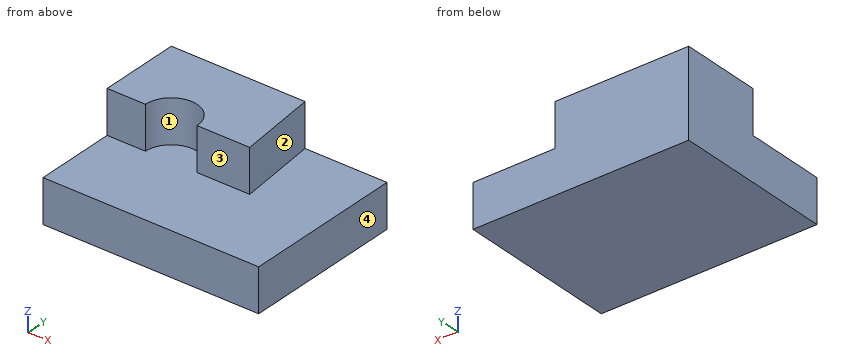
from build123d import *

# Parameters (mm, degrees)
F0_W     = 127
F0_H     = 95.25
F1_DEPTH = 25.4
F2_W     = 127
F2_H     = 47.6253371388
F3_DEPTH = 25.4
F5_DEPTH = 25.4


with BuildPart() as f1:
    # F0 (on Top) → F1 (new body)
    with BuildSketch(Plane.XY):
        Rectangle(F0_W, F0_H)
    extrude(amount=F1_DEPTH)

    # F2 (on face) → F3 (join)
    with BuildSketch(Plane.XY.offset(25.4)):
        with Locations((0, 23.8123314306)):
            Rectangle(F2_W, F2_H)
    extrude(amount=F3_DEPTH)

    # F4 (on face) → F5 (cut)
    with BuildSketch(Plane.XY.offset(50.8)):
        with BuildLine():
            Line((-40.9172700879, -0.0003371388), (-10.551281071, -0.0003371388))
            ThreePointArc((-10.551281071, -0.0003371388), (-25.7342755795, 15.1826573697), (-40.9172700879, -0.0003371388))
        make_face()
        Polygon((63.5, 47.625), (15.2478702366, 47.625), (20.4385407269, -0.0003371388), (63.5, -0.0003371388), align=None)
    extrude(amount=-F5_DEPTH, mode=Mode.SUBTRACT)


solid = f1.part
Build history of the part. All positions in model axes, mm. Face numbers are marked on the shaded views. A direction names the side the tool comes from. Coordinates: 2 decimals unless noted, no trailing zeros. Write each loop counter-clockwise with the first axis right and the second up, starting at its lowest first coordinate (ties: lowest second). Pieces come first, ordered by that corner, then holes.
(1) Pin check, flat tips, straight feed: pin 1 Ø3 at (x, z) = (-48.5, 42.5) entering from -Y; pin 2 Ø12 at (x, y) = (-24, -27) entering from -Z; pin 3 Ø6 at (x, y) = (25.5, -32.5) entering from +Z. Stop position of each tip, or through.
(2) Cut at C-C on y = 4.5. List the corners of the cut face in (x, z), and give its area (3 significant figures).
(3) 3-axis set-ups, long thin cutter, end or side, ignore diameter. For the marked faces 1, 2, 3 and 4: which of +Z, -Z, +X, -X, +Y, -Y reach the whole face in a straight line?
(4) Cut at B-B on z = 36. List the corners of the cut face in (x, y) (3 decimals), and give its area (3 significant figures).
(5) Cut at A-A on x = -48.5. List the corners of the cut face in (y, z) (3 decimals), and give its area (3 significant figures).
(6) Drill centre lines: line 1 (Z direction, x = -27.5, y = -12.5); line 2 (Y direction, x = -42.5, z = 38) (3 decimals); line 3 (X direction, y = 38, z = 31.5). Where is each one in solid material? Low to high.
(7) Cut at D-D on x = 25.5. List the corners of the cut face in (y, z) (3 decimals), and give its area (3 significant figures).
Working result:
1. pin 1: stops at y = 0
1. pin 2: stops at z = 0
1. pin 3: stops at z = 25.4
2. outline: (-63.5, 0) - (63.5, 0) - (63.5, 25.4) - (19.95, 25.4) - (19.95, 50.8) - (-11.23, 50.8) - (-11.23, 25.4) - (-40.23, 25.4) - (-40.23, 50.8) - (-63.5, 50.8) - close
2. area: 4,610 mm2
3. face 1: +Z, -Y
3. face 2: +Z, +X, +Y
3. face 3: +Z, +X, -X, -Y
3. face 4: +Z, -Z, +X, +Y, -Y
4. outline: (-63.5, 0) - (-40.917, 0) arc R15.183 cw to (-10.551, 0) - (20.439, 0) - (15.248, 47.625) - (-63.5, 47.625) - close
4. area: 3,510 mm2
5. outline: (-47.625, 0) - (47.625, 0) - (47.625, 50.8) - (0, 50.8) - (0, 25.4) - (-47.625, 25.4) - close
5. area: 3,630 mm2
6. line 1: z = 0 to 25.4
6. line 2: y = 0 to 47.625
6. line 3: x = -63.5 to 16.3
7. outline: (-47.625, 0) - (47.625, 0) - (47.625, 25.4) - (-47.625, 25.4) - close
7. area: 2,420 mm2
